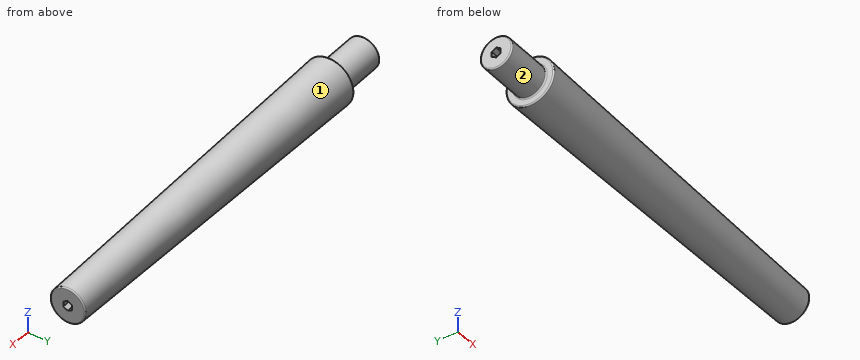
```python
from build123d import *

# Parameters (mm, degrees)
F0_W     = 59.7408
F0_H     = 31.75
F3_DEPTH = 821.767453
F4_R     = 2.54


with BuildPart() as f1:
    # F0 (on Front) → F1 (revolve)
    with BuildSketch(Plane.XZ):
        with Locations((-381.012826, 15.875)):
            Rectangle(F0_W, F0_H)
        Polygon((-351.142426, 31.75), (-351.142426, 0), (410.883226, 0), (410.883226, 34.925), (-317.004826, 47.625), (-317.004826, 31.75), align=None)
    revolve(axis=Axis((0, 0, 0), (1, 0, 0)))

    # F2 (on face) → F3 (cut, through all)
    with BuildSketch(Plane(origin=(-410.883226, 0, 0), x_dir=(0, -1, 0), z_dir=(-1, 0, 0))):
        Polygon((0, 10.081979), (-8.73125, 5.04099), (-8.73125, -5.04099), (0, -10.081979), (8.73125, -5.04099), (8.73125, 5.04099), align=None)
    extrude(amount=-F3_DEPTH, mode=Mode.SUBTRACT)

    # F4
    f4_edges = [f1.edges().sort_by_distance(p)[0] for p in [
        (-317.004826, 0, -47.625),
        (-410.883226, 0, -31.75),
        (410.883226, 0, -34.925),
        (-317.004826, 0, -31.75),
    ]]
    fillet(f4_edges, radius=F4_R)


solid = f1.part
```
Read the model definition and answer for the solid it produces. Units are mm, in the model's axes. Face numbers are marked on the shaded views. A direction names the side the tool comes from. Give positions to 0.01 mm unless a question says otherwise; leave off trailing zeros. Loops run counter-clockwise (first coordinate to the right, second up) from the corner with the lowest first, then second, coordinate; pieces in that order, holes last.
Item 1: The part is cut by section B-B (x = 113). Write down the section's boundary in (y, z).
Item 2: Each of these flat-tipped pins is pushed along its axis until it touches: pin 1 Ø8 at (x, z) = (175, 13.5) entering from -Y; pin 2 Ø8 at (x, z) = (-242.5, -14) entering from -Y; pin 3 Ø2 at (x, z) = (-205, -11) entering from -Y. Where does it stop, or does it pass through?
Item 3: For the marked faces 1 and 2, determine the directions among +Z, -Z, +X, -X, +Y, -Y from which every point of the face is accessible in a straight line to the end or side of a thin tool.
Item 4: The part is cut by section A-A (x = 319.5). Write down the section's boundary in (y, z), and give its area (3 significant figures).
Item 5: Find the intervals of material crossed by line 1 along Z through (x, y) = (-192.5, 32.5); line 2 along Y through (x, z) = (276, 23); line 3 along Y through (x, z) = (-70, 3), in increasing order.
Taken from the geometry:
1. outline: circle Ø80.24 at (0, 0); hole (-8.73, -5.04) - (0, -10.08) - (8.73, -5.04) - (8.73, 5.04) - (0, 10.08) - (-8.73, 5.04) - close
2. pin 1: stops at y = -37.87
2. pin 2: stops at y = -45.24
2. pin 3: stops at y = -44.56
3. face 1: +X
3. face 2: -X
4. outline: circle Ø73.04 at (0, 0); hole (-8.73, -5.04) - (0, -10.08) - (8.73, -5.04) - (8.73, 5.04) - (0, 10.08) - (-8.73, 5.04) - close
4. area: 3,930 mm2
5. line 1: z = -31.78 to 31.78
5. line 2: y = -29.34 to 29.34
5. line 3: y = -43.21 to -8.73, 8.73 to 43.21
